Can you work these out from the model? Positions are in its coordinate system, mm. A direction names the side the tool comes from. Coordinates: 2 decimals unless noted, no trailing zeros. Order: outer loops, then holes, each group sorted by start corner. A loop starts at its lowest first (then second) coordinate and runs counter-clockwise, first axis right, second up. Notation, with made-up numbers: (33.25, -38.5) -> (72.25, -38.5) arc R24 ccw to (72.25, -25.5) -> close; hole circle Ø5 at (15, 9.5). An arc over 180 degrees is marked (long way). Answer in a Markdown table with one row per item.
```python
from build123d import *

# Parameters (mm, degrees)
F1_DEPTH    = 15.7
F2_W        = 10.0960650777
F2_H        = 2.9
F3_DEPTH    = 8
F4_R        = 5
F5_T1_DEPTH = 26.8923143391
F5_T3_DEPTH = 21.3473434867
F5_T5_DEPTH = 35.7
F6_W        = 15
F6_H        = 6.25
F7_DEPTH    = 2
F8_SIZE     = 1.99999


# Not quite as in the source:
# - a fillet or chamfer that OpenCascade refuses, or shapes differently, is made with other operations: its cross-section is extruded or revolved along the edge and cut away or added
# - a fillet or chamfer is up to 0.001 mm smaller than in the source, because OpenCascade refuses the exact size


with BuildPart() as f1:
    # F0 (on Top) → F1 (new body)
    with BuildSketch(Plane.XY):
        Polygon((30, 9), (0, 9), (0, -1.8), (15, -1.8), (15, -9), (19.5954625243, -9), (30, -2.6151265483), align=None)
        with BuildLine():
            ThreePointArc((21.17, -5.2), (17.9264971157, -6.5435028843), (19.27, -3.3))
            ThreePointArc((19.27, -3.3), (20.6135028843, -3.8564971157), (21.17, -5.2))
        make_face(mode=Mode.SUBTRACT)
        with BuildLine():
            ThreePointArc((19.27, 3.9), (17.9264971157, 7.1435028843), (21.17, 5.8))
            ThreePointArc((21.17, 5.8), (20.6135028843, 4.4564971157), (19.27, 3.9))
        make_face(mode=Mode.SUBTRACT)
        with BuildLine():
            ThreePointArc((24.47, 5.8), (26.37, 7.7), (28.27, 5.8))
            ThreePointArc((28.27, 5.8), (26.37, 3.9), (24.47, 5.8))
        make_face(mode=Mode.SUBTRACT)
    extrude(amount=F1_DEPTH)

    # F2 (on face) → F3 (cut)
    with BuildSketch(Plane.XY.offset(15.7)):
        with BuildLine():
            ThreePointArc((11.6039349223, 0.5750306588), (9.4802536205, 3.5683191144), (13.0070529624, 4.5839393448))
            Line((13.0070529624, 4.5839393448), (16.2772942688, 1.9751998411))
            ThreePointArc((16.2772942688, 1.9751998411), (16.3347359589, 2.3983908199), (16.3539349223, 2.8250306588))
            ThreePointArc((16.3539349223, 2.8250306588), (16.0161356009, 4.5842876531), (15.050783271, 6.09332325))
            ThreePointArc((15.050783271, 6.09332325), (7.4840088208, 5.1890756918), (10.5215341623, -1.8))
            Line((10.5215341623, -1.8), (12.6863356823, -1.8))
            ThreePointArc((12.6863356823, -1.8), (14.4922032842, -0.9459646832), (15.787235055, 0.5750306588))
            Line((15.787235055, 0.5750306588), (11.6039349223, 0.5750306588))
        make_face()
        with BuildLine():
            ThreePointArc((16.3539349223, 2.8250306588), (16.3347359589, 2.3983908199), (16.2772942688, 1.9751998411))
            Line((16.2772942688, 1.9751998411), (16.9157389312, 1.4658992557))
            ThreePointArc((16.9157389312, 1.4658992557), (17.0544357572, 1.2919384682), (17.1039349223, 1.0750306588))
            ThreePointArc((17.1039349223, 1.0750306588), (16.9574883129, 0.7214772682), (16.6039349223, 0.5750306588))
            Line((16.6039349223, 0.5750306588), (15.787235055, 0.5750306588))
            ThreePointArc((15.787235055, 0.5750306588), (14.4922032842, -0.9459646832), (12.6863356823, -1.8))
            Line((12.6863356823, -1.8), (15, -1.8))
            Line((15, -1.8), (15, -1.9249693412))
            Line((15, -1.9249693412), (19.9039349223, -1.9249693412))
            Line((19.9039349223, -1.9249693412), (19.9039349223, 0.9750306588))
            Line((19.9039349223, 0.9750306588), (15.050783271, 6.09332325))
            ThreePointArc((15.050783271, 6.09332325), (16.0161356009, 4.5842876531), (16.3539349223, 2.8250306588))
        make_face()
        with Locations((24.9519674612, -0.4749693412)):
            Rectangle(F2_W, F2_H)
    extrude(amount=-F3_DEPTH, mode=Mode.SUBTRACT)

    # F4
    f4_edges = [f1.edges().sort_by_distance(p)[0] for p in [
        (19.903935, 0.975031, 11.7),
    ]]
    fillet(f4_edges, radius=F4_R)

    # F5: fillet of radius 4 on 4 edges, made by hand

    # F5_s2 → F5_t1 (cut)
    with BuildSketch(Plane.XY.offset(-5.5961571696)):
        with BuildLine():
            ThreePointArc((30, -0.3766636805), (29.4905957559, -2.3300559271), (28.0921293656, -3.7859150232))
            Line((28.0921293656, -3.7859150232), (30, -2.6151265483))
            Line((30, -2.6151265483), (30, -0.3766636805))
        make_face()
    extrude(amount=F5_T1_DEPTH, mode=Mode.SUBTRACT)

    # F5_s4 → F5_t3 (cut)
    with BuildSketch(Plane.XY.offset(-2.8236717433)):
        with BuildLine():
            ThreePointArc((20.5581231925, -8.4092513427), (19.5529608525, -8.8494808332), (18.465993827, -9))
            Line((18.465993827, -9), (19.5954625243, -9))
            Line((19.5954625243, -9), (20.5581231925, -8.4092513427))
        make_face()
    extrude(amount=F5_T3_DEPTH, mode=Mode.SUBTRACT)

    # F5_s6 → F5_t5 (cut)
    with BuildSketch(Plane.XY.offset(-10)):
        with BuildLine():
            ThreePointArc((15, -5), (16.1715728753, -7.8284271247), (19, -9))
            Line((19, -9), (15, -9))
            Line((15, -9), (15, -5))
        make_face()
        with BuildLine():
            ThreePointArc((30, 5), (28.8284271247, 7.8284271247), (26, 9))
            Line((26, 9), (30, 9))
            Line((30, 9), (30, 5))
        make_face()
    extrude(amount=F5_T5_DEPTH, mode=Mode.SUBTRACT)

    # F6 (on face) → F7 (cut)
    with BuildSketch(Plane.XZ.offset(1.8)):
        with Locations((7.5, 3.125)):
            Rectangle(F6_W, F6_H)
    extrude(amount=-F7_DEPTH, mode=Mode.SUBTRACT)

    # F8 (size 2 in the source; OpenCascade refuses exactly that, so slightly less here)
    f8_edges = [f1.edges().sort_by_distance(p)[0] for p in [
        (7.5, 0.2, 6.25),
    ]]
    chamfer(f8_edges, length=F8_SIZE)

    # F9: F1 across plane


with BuildPart() as f1_1:
    add(f1.part)
    add(f1.part.mirror(Plane.YZ))


solid = f1_1.part
```
(1) On a 3-axis mill with a long thin cutter (end or side, diameter ignored), from which of +Z, -Z, +X, -X, +Y, -Y can I reach the whole of each face in a straight line? I mean faces 1 (the flat face through (-18, 2, 7.7)), 2 (the flat face through (-22, -1.925, 12)), 3 (the flat face through (14, 0.575, 12)), 4 (the cylindrical face through (-16.05, -7.7, 7.74)), 5 (the flat face through (0, 0.2, 2)). Say none if no direction works.
Response values:
| item | result |
|---|---|
| face 1 | +Z |
| face 2 | +Z, +X, -X |
| face 3 | +Z, +X |
| face 4 | +Z, -Z, -Y |
| face 5 | -Z, -Y |
(2) I need wall thicknesses on line 1 (X direction, y = -3.5, z = 10.5); line 2 (X direction, y = -0.5, z = 3); line 3 (X direction, y = 5.8, z = 5.75). Which ranges of each line are inside material? Lowest first, please. Write a range as [from, to].
Response values:
| item | result |
|---|---|
| line 1 | [-28.5, -20.12], [-18.42, -15], [15, 18.42], [20.12, 28.5] |
| line 2 | [-30, -15], [15, 30] |
| line 3 | [-29.92, -28.27], [-24.47, -21.17], [-17.37, 17.37], [21.17, 24.47], [28.27, 29.92] |
(3) Suppose I cut it at B-B (y = -6.5). Please give me the cut outline in (x, z).
Response values:
| item | result |
|---|---|
| outline | (-23.67, 0) -> (-20.66, 0) -> (-20.66, 15.7) -> (-23.67, 15.7) -> close; (-17.88, 0) -> (-15.29, 0) -> (-15.29, 15.7) -> (-17.88, 15.7) -> close; (15.29, 0) -> (17.88, 0) -> (17.88, 15.7) -> (15.29, 15.7) -> close; (20.66, 0) -> (23.67, 0) -> (23.67, 15.7) -> (20.66, 15.7) -> close |
(4) Will these pins go through, and if not, where does the flat tip stop? pin 1 Ø1.6 at (y, z) = (-2.5, 4.5) entering from -X; pin 2 Ø3 at (y, z) = (-3, 12.5) entering from +X; pin 3 Ø4 at (x, z) = (25, 11) entering from -Y; pin 4 Ø2.5 at (x, y) = (19.27, 5.8) entering from -Z.
Response values:
| item | result |
|---|---|
| pin 1 | x = -29.77 |
| pin 2 | x = 29.69 |
| pin 3 | y = -6.91 |
| pin 4 | through |
(5) Suppose I cut it at A-A (z = 3.25). Please give me the cut outline in (x, y).
Response values:
| item | result |
|---|---|
| outline | (-30, -0.38) arc R4 ccw to (-28.09, -3.79) -> (-20.56, -8.41) arc R4 ccw to (-18.73, -8.99) arc R4 ccw to (-15, -5) -> (-15, 0.2) -> (15, 0.2) -> (15, -5) arc R4 ccw to (18.73, -8.99) arc R4 ccw to (20.56, -8.41) -> (28.09, -3.79) arc R4 ccw to (30, -0.38) -> (30, 5) arc R4 ccw to (26, 9) -> (-26, 9) arc R4 ccw to (-30, 5) -> close; hole circle Ø3.8 at (-26.37, 5.8); hole circle Ø3.8 at (-19.27, -5.2); hole circle Ø3.8 at (-19.27, 5.8); hole circle Ø3.8 at (19.27, -5.2); hole circle Ø3.8 at (19.27, 5.8); hole circle Ø3.8 at (26.37, 5.8) |
(6) Suppose I cut it at C-C (y = 3.25). Please give me the cut outline in (x, z).
Response values:
| item | result |
|---|---|
| outline | (-30, 0) -> (30, 0) -> (30, 15.7) -> (17.75, 15.7) -> (17.75, 7.7) -> (14.68, 7.7) -> (14.68, 15.7) -> (9.39, 15.7) -> (9.39, 7.7) -> (6.87, 7.7) -> (6.87, 15.7) -> (-6.87, 15.7) -> (-6.87, 7.7) -> (-9.39, 7.7) -> (-9.39, 15.7) -> (-14.68, 15.7) -> (-14.68, 7.7) -> (-17.75, 7.7) -> (-17.75, 15.7) -> (-30, 15.7) -> close |
(7) We'd pull the mould along Y, two halves only. Please class faces 6 (the flat face through (22, -1.925, 12)), 7 (the cylindrical face through (28.859, 7.797, 7.74)), 8 (the flat face through (24.27, -6.13, 7.74)): +Y half, -Y half, draft (parallel to the pull), parting line (faces both ways), or undercut.
Response values:
| item | result |
|---|---|
| face 6 | undercut |
| face 7 | +Y half |
| face 8 | -Y half |
